```python
from build123d import *

# Parameters (mm, degrees)
SKETCH1_R           = 11.45
BOSS_EXTRUDE1_DEPTH = 4
SKETCH2_R           = 10
BOSS_EXTRUDE2_DEPTH = 4
SKETCH3_R           = 4
CUT_EXTRUDE1_DEPTH  = 8
CHAMFER1_SIZE       = 0.5


with BuildPart() as part:
    # Sketch1 → Boss-Extrude1 (new body)
    with BuildSketch(Plane(origin=(0, 0, 0), x_dir=(0, 0, -1), z_dir=(1, 0, 0))):
        Circle(SKETCH1_R)
    extrude(amount=BOSS_EXTRUDE1_DEPTH)

    # Sketch2 → Boss-Extrude2 (add)
    with BuildSketch(Plane(origin=(4, 0, 0), x_dir=(0, 0, -1), z_dir=(1, 0, 0))):
        Circle(SKETCH2_R)
    extrude(amount=BOSS_EXTRUDE2_DEPTH)

    # Sketch3 → Cut-Extrude1 (cut)
    with BuildSketch(Plane(origin=(8, 0, 0), x_dir=(0, 0, -1), z_dir=(1, 0, 0))):
        Circle(SKETCH3_R)
    extrude(amount=-CUT_EXTRUDE1_DEPTH, mode=Mode.SUBTRACT)

    # Chamfer1
    chamfer1_edges = [part.edges().sort_by_distance(p)[0] for p in [
        (0, 0, 4),
        (8, 0, 10),
    ]]
    chamfer(chamfer1_edges, length=CHAMFER1_SIZE)


solid = part.part
```
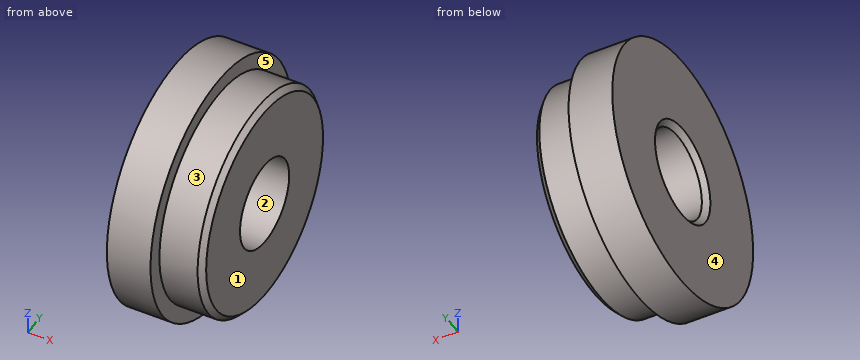
For this review, take the finished solid that the model builds, in its own axes (mm). Face numbers are marked on the shaded views. A direction names the side the tool comes from. Give positions to 0.01 mm unless a question says otherwise; leave off trailing zeros. Write each loop counter-clockwise with the first axis right and the second up, starting at its lowest first coordinate (ties: lowest second). Pieces come first, ordered by that corner, then holes. Notation, with made-up numbers: M 66.5,87 L 120.5,87 A20 cw 120.5,112 Z; hole C 51.25,71.5 d2. An arc over 180 degrees is marked long. Answer as a JSON object with one key per item and string values. Group by question number.
Item 1: Draft analysis for pull direction Z (two halves, no side actions). For the marked faces 1, 2 and 3, state which applies: +Z half, -Z half, draft (parallel to the pull), parting line (faces both ways), or undercut.
Item 2: Consider section C-C on x = 2. Write out the cut boundary in (y, z), plus the area to 3 significant figures.
Item 3: For pin 1 Ø3 at (x, z) = (2.5, -6) entering from +Y; pin 2 Ø1.5 at (y, z) = (8.5, 6.5) entering from +X; pin 3 Ø3 at (y, z) = (-8.5, -2) entering from -X; pin 4 Ø7 at (y, z) = (0, 0) entering from -X, all flat-tipped, find the tip position at first contact; note any pin that passes through.
Item 4: Tool access review of the marked faces 4 and 5: name each direction out of +Z, -Z, +X, -X, +Y, -Y from which nothing blocks a thin tool from reaching the whole face with its end or side.
Item 5: For probe 1 along Y at (x, z) = (3.5, 0); probe 2 along X at (y, z) = (3, 10); probe 3 along Y at (x, z) = (5.5, -2), list the stretches that pass through material, from the lowest coordinate up. Write a range as [from, to].
Item 6: Consider section D-D on x = 7. Write out the cut boundary in (y, z), plus the area to 3 significant figures.
Item 7: Consider section A-A on z = 0. Write out the cut boundary in (x, y), plus the area to 3 significant figures.
Check result:
{
 "1": {"face 1": "draft", "face 2": "undercut", "face 3": "parting line"},
 "2": {"outline": "C 0,0 d22.9; hole C 0,0 d8", "area": "362 mm^2"},
 "3": {"pin 1": "stops at y = 10.53", "pin 2": "stops at x = 7.55", "pin 3": "stops at x = 0", "pin 4": "passes through"},
 "4": {"face 4": "+Z, -Z, -X, +Y, -Y", "face 5": "+X"},
 "5": {"probe 1": "y = [-11.45, -4], [4, 11.45]", "probe 2": "x = [0, 4]", "probe 3": "y = [-9.8, -3.46], [3.46, 9.8]"},
 "6": {"outline": "C 0,0 d20; hole C 0,0 d8", "area": "264 mm^2"},
 "7": {"outline": "M 0,-11.45 L 4,-11.45 L 4,-10 L 7.5,-10 L 8,-9.5 L 8,-4 L 0.5,-4 L 0,-4.5 Z; M 0,4.5 L 0.5,4 L 8,4 L 8,9.5 L 7.5,10 L 4,10 L 4,11.45 L 0,11.45 Z", "area": "107 mm^2"}
}
